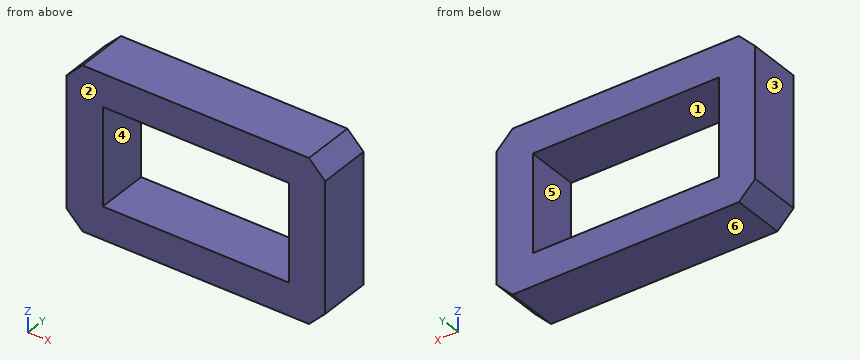
```python
from build123d import *

# Parameters (mm, degrees)
SKETCH1_W           = 32
SKETCH1_H           = 20
BOSS_EXTRUDE1_DEPTH = 6.5
SKETCH2_W           = 23
SKETCH2_H           = 12
CUT_EXTRUDE1_DEPTH  = 20.956202043
CHAMFER1_SIZE       = 2


with BuildPart() as part:
    # Sketch1 → Boss-Extrude1 (new body)
    with BuildSketch(Plane(origin=(0, 0, 0), x_dir=(1, 0, 0), z_dir=(0, 1, 0))):
        Rectangle(SKETCH1_W, SKETCH1_H)
    extrude(amount=BOSS_EXTRUDE1_DEPTH)

    # Sketch2 → Cut-Extrude1 (cut, through all)
    with BuildSketch(Plane(origin=(0, 6.5, 0), x_dir=(1, 0, 0), z_dir=(0, 1, 0))):
        Rectangle(SKETCH2_W, SKETCH2_H)
    extrude(amount=-CUT_EXTRUDE1_DEPTH, mode=Mode.SUBTRACT)

    # Chamfer1
    chamfer1_edges = [part.edges().sort_by_distance(p)[0] for p in [
        (16, 3.25, 10),
        (-16, 3.25, 10),
        (-16, 3.25, -10),
        (16, 3.25, -10),
    ]]
    chamfer(chamfer1_edges, length=CHAMFER1_SIZE)


solid = part.part
```
Source: CAD feature listing. Evaluate the final solid. Frame: model axes, mm. Face numbers are marked on the shaded views. A direction names the side the tool comes from. Give positions to 0.01 mm unless a question says otherwise; leave off trailing zeros. Write each loop counter-clockwise with the first axis right and the second up, starting at its lowest first coordinate (ties: lowest second). Pieces come first, ordered by that corner, then holes. Notation, with made-up numbers: (52, -16.5) - (108, -16.5) arc R27 ccw to (108, 2.5) - close; hole circle Ø11 at (72.25, 3.25). An arc over 180 degrees is marked (long way). One line per item, written item: value. Start each with the question number.
Q1. Section query C-C, the plane z = -5. Return the cut outline in (x, y), then the cut area to 3 significant figures.
Q2. Section query A-A, the plane x = 5. Return the cut outline in (y, z).
Q3. Material intervals for probe 1 along Z at (x, y) = (-7, 1.25); probe 2 along X at (y, z) = (3, 4); probe 3 along X at (y, z) = (2, 9.25), sorted ascending. Write a range as from..to.
Q4. Draft query along Z for the marked faces 3, 4, 5 and 6. Return one class per face: +Z half, -Z half, draft (parallel to the pull), parting line (faces both ways), or undercut.
Q5. Set-up query: the marked faces 1 and 2. Return all of +Z, -Z, +X, -X, +Y, -Y with unobstructed straight access to the full face (end or side cutting, diameter ignored); none if empty.
Q6. Section query B-B, the plane y = 5. Return the cut outline in (x, z), then the cut area to 3 significant figures.
Answer:
1. outline: (-16, 0) - (-11.5, 0) - (-11.5, 6.5) - (-16, 6.5) - close; (11.5, 0) - (16, 0) - (16, 6.5) - (11.5, 6.5) - close
1. area: 58.5 mm2
2. outline: (0, -10) - (6.5, -10) - (6.5, -6) - (0, -6) - close; (0, 6) - (6.5, 6) - (6.5, 10) - (0, 10) - close
3. probe 1: z = -10..-6, 6..10
3. probe 2: x = -16..-11.5, 11.5..16
3. probe 3: x = -14.75..14.75
4. face 3: draft
4. face 4: undercut
4. face 5: undercut
4. face 6: -Z half
5. face 1: +Y, -Y
5. face 2: +Z, -Z, +X, -X, -Y
6. outline: (-16, -8) - (-14, -10) - (14, -10) - (16, -8) - (16, 8) - (14, 10) - (-14, 10) - (-16, 8) - close; hole (-11.5, -6) - (11.5, -6) - (11.5, 6) - (-11.5, 6) - close
6. area: 356 mm2
